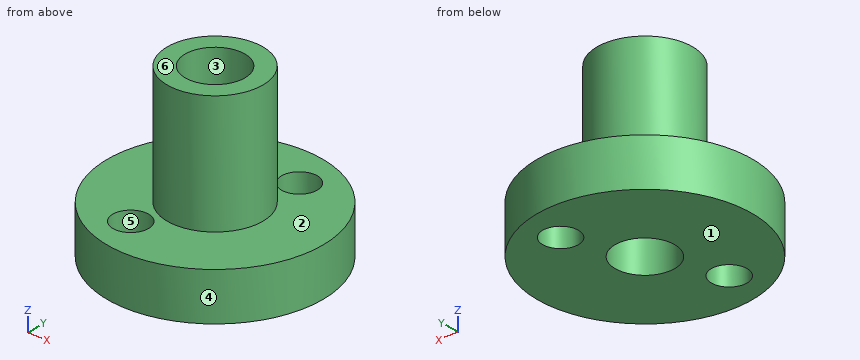
```python
from build123d import *

# Parameters (mm, degrees)
SKETCH_1_R               = 18
SKETCH_1_R_2             = 5
EXTRUDE_1_DEPTH          = 8
SKETCH_2_R               = 8
SKETCH_2_R_2             = 5
EXTRUDE_2_DEPTH          = 20
SKETCH_3_R               = 3
CUT_EXTRUDE_1_DEPTH      = 20
PATTERN_CIRCULAR_1_COUNT = 2


with BuildPart() as part:
    # Эскиз1 → Бобышка-Вытянуть1 (new body)
    with BuildSketch(Plane.XY):
        Circle(SKETCH_1_R)
        Circle(SKETCH_1_R_2, mode=Mode.SUBTRACT)
    extrude(amount=EXTRUDE_1_DEPTH)

    # Эскиз2 → Бобышка-Вытянуть2 (add)
    with BuildSketch(Plane.XY.offset(8)):
        Circle(SKETCH_2_R)
        Circle(SKETCH_2_R_2, mode=Mode.SUBTRACT)
    extrude(amount=EXTRUDE_2_DEPTH)

    # Эскиз3 → Вырез-Вытянуть1 (cut)
    with BuildSketch(Plane(origin=(0, 0, 0), x_dir=(-1, 0, 0), z_dir=(0, 0, -1))):
        with Locations((5.029540605, -10.89512374)):
            Circle(SKETCH_3_R)
    cut_extrude_1 = extrude(amount=-CUT_EXTRUDE_1_DEPTH, mode=Mode.SUBTRACT)

    # Круговой массив1: Вырез-Вытянуть1 ×2 about axis
    pattern_circular_1_axis = Axis((0, 0, 0), (0, 0, 1))
    for i in range(1, PATTERN_CIRCULAR_1_COUNT):
        add(cut_extrude_1.rotate(pattern_circular_1_axis, i * 360 / PATTERN_CIRCULAR_1_COUNT), mode=Mode.SUBTRACT)


solid = part.part
```
The model under review builds one solid part; all positions refer to its coordinate system, in mm. Face numbers are marked on the shaded views. A direction names the side the tool comes from. Give positions to 0.01 mm unless a question says otherwise; leave off trailing zeros. Write each loop counter-clockwise with the first axis right and the second up, starting at its lowest first coordinate (ties: lowest second). Pieces come first, ordered by that corner, then holes. Notation, with made-up numbers: M 18.25,-24 L 30.25,-24 A15 cw 30.25,-2 Z; hole C 37.5,62 d3. An arc over 180 degrees is marked long. Write each question's results on one line, items separated by ' | '. Start each with the question number.
1. We need section A-A (y = 0). Write out the cut boundary in (x, z).
2. Insertion check: pin 1 Ø2 at (x, z) = (-8, 15) entering from +Y; pin 2 Ø2 at (x, y) = (-11, 12) entering from +Z; pin 3 Ø6 at (y, z) = (6, 6.5) entering from -X. Each pin has a flat end and moves straight along its axis. Give the tip position at first contact, or say it passes through.
3. For the marked faces 1 and 2, list the 3-axis set-ups (+Z, -Z, +X, -X, +Y, -Y) from which the entire face can be reached by the end or side of a thin tool; tool diameter is ignored.
4. We need section D-D (z = 13). Write out the cut boundary in (x, y), and give its area (3 significant figures).
5. For probe 1 along Y at (x, z) = (4.5, 4.5); probe 2 along Y at (x, z) = (0, 10.5); probe 3 along Z at (x, y) = (12, 12), list the stretches that pass through material, from the lowest coordinate up. Write a range as [from, to].
6. Mouldability with a two-part tool opening along X and no side actions: class the marked faces 3, 4, 5 and 6 as released by +X, released by -X, zero draft, split by the parting line, or undercut.
7. We need section C-C (y = 9). Write out the cut boundary in (x, z), and give its area (3 significant figures).
Results found:
1) outline: M -18,0 L -5,0 L -5,28 L -8,28 L -8,8 L -18,8 Z; M 5,0 L 18,0 L 18,8 L 8,8 L 8,28 L 5,28 Z
2) pin 1: stops at y = 3.87 | pin 2: stops at z = 8 | pin 3: stops at x = -17.75
3) face 1: -Z, +X, -X, +Y, -Y | face 2: +Z
4) outline: C 0,0 d16; hole C 0,0 d10 | area: 123 mm^2
5) probe 1: y = [-17.43, -2.18], [2.18, 7.94], [13.85, 17.43] | probe 2: y = [-8, -5], [5, 8] | probe 3: z = [0, 8]
6) face 3: undercut | face 4: split by the parting line | face 5: undercut | face 6: zero draft
7) outline: M -15.59,0 L 2.7,0 L 2.7,8 L -15.59,8 Z; M 7.36,0 L 15.59,0 L 15.59,8 L 7.36,8 Z | area: 212 mm^2
